Geometry check sheet. Reference: the model listing, model coordinates, mm. A direction names the side the tool comes from. Give positions to 0.01 mm unless a question says otherwise; leave off trailing zeros. Loops run counter-clockwise (first coordinate to the right, second up) from the corner with the lowest first, then second, coordinate; pieces in that order, holes last. Notation, with made-up numbers: (12, -28) -> (56, -28) arc R18 ccw to (56, -4) -> close; hole circle Ø10 at (12.5, -3). An arc over 180 degrees is marked (long way). Answer as a JSON object with one key per item and string values.
from build123d import *

# Parameters (mm, degrees)
F1_DEPTH = 5.08
F2_T     = -2.54
F3_W     = 3.9589210415
F3_H     = 12.6681532711
F3_W_2   = 146.1344220674
F4_DEPTH = 1.778
F6_DEPTH = 1.778
F7_SIZE  = 12.7
F8_SIZE  = 25.39999


# Not quite as in the source:
# - a fillet or chamfer is up to 0.001 mm smaller than in the source, because OpenCascade refuses the exact size


with BuildPart() as f1:
    # F0 (on Front) → F1 (new body)
    with BuildSketch(Plane.XZ):
        Polygon((104.074490943, -25.4), (104.074490943, 25.4), (-20.8395591676, 25.4), (-20.8395591676, 15.409566462), (-66.9992624521, 15.409566462), (-66.9992624521, 25.4), (-99.125509057, 25.4), (-99.125509057, -25.4), align=None)
    extrude(amount=F1_DEPTH)

    # F2
    f2_openings = [f1.faces().sort_by_distance(p)[0] for p in [
        (4.64404, -5.08, -0.954203),
    ]]
    offset(amount=F2_T, openings=f2_openings, kind=Kind.INTERSECTION)

    # F3 (on face) → F4 (join)
    with BuildSketch(Plane(origin=(0, 0, 0), x_dir=(-1, 0, 0), z_dir=(0, 1, 0))):
        with Locations((101.1049695778, 6.3340766355)):
            Rectangle(F3_W, F3_H)
        with Locations((26.0582980233, 6.3340766355)):
            Rectangle(F3_W_2, F3_H)
    extrude(amount=F4_DEPTH)

    # F5 (on face) → F6 (join)
    with BuildSketch(Plane(origin=(0, 0, 0), x_dir=(-1, 0, 0), z_dir=(0, 1, 0))):
        Polygon((-47.0089130104, 12.6681532711), (-47.0089130104, 25.4), (-104.074490943, 25.4), (-104.074490943, -25.4), (-47.0089130104, -25.4), (-47.0089130104, 0), align=None)
    extrude(amount=F6_DEPTH)

    # F7
    f7_edges = [f1.edges().sort_by_distance(p)[0] for p in [
        (47.008913, 0.889, 25.4),
    ]]
    chamfer(f7_edges, length=F7_SIZE)

    # F8 (size 25.4 in the source; OpenCascade refuses exactly that, so slightly less here)
    f8_edges = [f1.edges().sort_by_distance(p)[0] for p in [
        (47.008913, 0.889, -25.4),
    ]]
    chamfer(f8_edges, length=F8_SIZE)


solid = f1.part
1) Section check A-A on x = 80.5. Record the cut outline in (y, z).
Geometry check:
{"outline": "(-5.08, -25.4) -> (1.78, -25.4) -> (1.78, 25.4) -> (-5.08, 25.4) -> (-5.08, 22.86) -> (-2.54, 22.86) -> (-2.54, -22.86) -> (-5.08, -22.86) -> close"}
2) Section check C-C on x = -75.5. Record the cut outline in (y, z), plus the area to 3 significant figures.
Geometry check:
{"outline": "(-5.08, -25.4) -> (0, -25.4) -> (0, 0) -> (1.78, 0) -> (1.78, 12.67) -> (0, 12.67) -> (0, 25.4) -> (-5.08, 25.4) -> (-5.08, 22.86) -> (-2.54, 22.86) -> (-2.54, -22.86) -> (-5.08, -22.86) -> close", "area": "164 mm2"}
3) Material ranges on line 1 along X through (y, z) = (-4.25, 19); line 2 along X through (y, z) = (-4, 11.5); line 3 along Z through (x, y) = (-42, -3.5), recorded low to high. Write a range as from..to.
Geometry check:
{"line 1": "x = -99.13..-96.59, -69.54..-67, -20.84..-18.3, 101.53..104.07", "line 2": "x = -99.13..-96.59, 101.53..104.07", "line 3": "z = -25.4..-22.86, 12.87..15.41"}
4) Section check D-D on z = -4. Record the cut outline in (x, y).
Geometry check:
{"outline": "(-99.13, -5.08) -> (-96.59, -5.08) -> (-96.59, -2.54) -> (101.53, -2.54) -> (101.53, -5.08) -> (104.07, -5.08) -> (104.07, 1.78) -> (51.01, 1.78) -> (51.01, 0) -> (-99.13, 0) -> close"}
5) Section check B-B on z = 5. Record the cut outline in (x, y), plus the area to 3 significant figures.
Geometry check:
{"outline": "(-103.08, 0) -> (-99.13, 0) -> (-99.13, -5.08) -> (-96.59, -5.08) -> (-96.59, -2.54) -> (101.53, -2.54) -> (101.53, -5.08) -> (104.07, -5.08) -> (104.07, 1.78) -> (-103.08, 1.78) -> close", "area": "897 mm2"}
6) Depth check by flat-ended pin: P1, Ø0.9, axis at x = -42, y = 0.5, coming from the +Z side; P2, Ø4, axis at y = -3.5, z = 9, coming from the -X side; P3, Ø12, axis at x = 51.5, z = -4, coming from the -Y side. Enter the tip coordinate at first touch or a pass-through.
Geometry check:
{"P1": "stops at z = 12.67", "P2": "stops at x = -99.13", "P3": "stops at y = -2.54"}
7) Tool access check on faces 1 (the face through (-66.999, -3, 20)), 2 (the face through (-15, 0, -13)), 3 (the face through (-21, 0, 15)). Record the directions out of +Z, -Z, +X, -X, +Y, -Y that give a thin tool (end or side, any length) a straight path to the whole face; none if there is none.
Geometry check:
{"face 1": "+Z, +Y, -Y", "face 2": "-Z, -X, +Y", "face 3": "+Z, -X, +Y"}
8) Draft check along X on faces 4 (the face through (-20.84, -3, 20)), 5 (the face through (-44, -3, 15.41)), 6 (the face through (53.27, 0.88, 18.96)), 7 (the face through (-101, 0, 6)). Enter one of: pulls with the +X half, pulls with the -X half, needs draft (parallel to the pull), parting line crosses it, or undercut.
Geometry check:
{"face 4": "undercut", "face 5": "undercut", "face 6": "pulls with the -X half", "face 7": "needs draft"}
